Read the model definition and answer for the solid it produces. Units are mm, in the model's axes. A direction names the side the tool comes from. Round coordinates to 2 decimals unless told otherwise and drop trailing zeros. Write each loop counter-clockwise with the first axis right and the second up, starting at its lowest first coordinate (ties: lowest second). Pieces come first, ordered by that corner, then holes. Notation, with made-up numbers: (-5, 48.25) -> (7, 48.25) arc R9 cw to (7, 54.25) -> close; hole circle Ø6 at (37, 13.5). An arc over 180 degrees is marked (long way). Return JSON: item names as keys, results as strings. Group by question number.
(1) The mould has two halves that part along Z. Classify faces 1 (the flat face through (0, -152.4, 5)), 2 (the flat face through (-6.096, -75, -50)), 3 (the cylindrical face through (0.219, -129.486, -143.179)): released by +Z, released by -Z, zero draft, split by the parting line, or undercut.
(2) A cutting plane is placed at C-C on x = -21. Give the vertices of the cut face in (y, z).
(3) For faces 4 (the flat face through (0, -75, 0.191)), 5 (the flat face through (15.621, -58, -54)), 6 (the cylindrical face through (0.114, -131.979, -82.357)), 7 (the flat face through (0, 0, 5)), 8 (the flat face through (-15.621, -58, -52)), determine the directions among +Z, -Z, +X, -X, +Y, -Y from which every point of the face is accessible in a straight line to the end or side of a thin tool.
(4) A cutting plane is placed at D-D on y = -130. Give the vertices of the cut face in (x, z), then the cut area to 3 significant figures.
(5) Given pin 1 (1.5 mm diameter, centred on x = -10.5, y = -62.5, fed in from +Z); pin 2 (4 mm diameter, centred on x = 20, y = -24, fed in from +Z); pin 3 (8 mm diameter, centred on x = -19, z = -138.5, fed in from +Y); pin 4 (15 mm diameter, centred on x = 0, z = 38.29, fed in from -Y), each flat-ended and moving along its own axis, determine where each tip first touches the part or whether it passes through.
(6) Straight lines are drawn through the part: line 1 (Y direction, x = 7, z = 16.5); line 2 (X direction, y = -89, z = -46); line 3 (Z direction, x = 6, y = -76). For each, find the intervals that lie inside material, in ascending order.
(7) A cutting plane is placed at B-B on x = -10. State how many separate pieces and enclosed holes the cut face has, then the cut area to 3 significant figures.
(8) A cutting plane is placed at A-A on z = -41.5. Give the vertices of the cut face in (x, y).
```python
from build123d import *

# Parameters (mm, degrees)
F0_R          = 12.7
F1_DEPTH      = 152.4
F2_R          = 76.19999
F3_W          = 101.6
F3_H          = 56.6531687857
F4_DEPTH      = 41.022
F4_DEPTH_BACK = 25.4
F6_DEPTH      = 152.401
F3_H_2        = 18.0714114576
F7_DEPTH      = 41.022
F3_R          = 38.1
F8_DEPTH      = 41.022


# Not quite as in the source:
# - a fillet or chamfer is up to 0.001 mm smaller than in the source, because OpenCascade refuses the exact size
# - a feature names something its author has since deleted; it is built from what else it names


with BuildPart() as f1:
    # F0 (on Front) → F1 (new body)
    with BuildSketch(Plane.XZ):
        with BuildLine():
            ThreePointArc((15.621, 18.2628701244), (22.8246949596, 27.1472538948), (25.4, 38.2914586668))
            ThreePointArc((25.4, 38.2914586668), (-11.144204772, 61.1161536264), (-15.621, 18.2628701244))
            ThreePointArc((-15.621, 18.2628701244), (0, 12.8914586668), (15.621, 18.2628701244))
        make_face()
        with Locations((0, 38.2914586668)):
            Circle(F0_R, mode=Mode.SUBTRACT)
        with BuildLine():
            ThreePointArc((15.621, 18.2628701244), (0, 12.8914586668), (-15.621, 18.2628701244))
            Line((-15.621, 18.2628701244), (-15.621, -164.9085413332))
            Line((-15.621, -164.9085413332), (15.621, -164.9085413332))
            Line((15.621, -164.9085413332), (15.621, 18.2628701244))
        make_face()
    extrude(amount=F1_DEPTH)

    # F2 (radius 76.2 in the source; OpenCascade refuses exactly that, so slightly less here)
    f2_edges = [f1.edges().sort_by_distance(p)[0] for p in [
        (0, -152.4, -164.908541),
        (0, 0, -164.908541),
    ]]
    fillet(f2_edges, radius=F2_R)

    # F3 (on face) → F4 (cut, two sides)
    with BuildSketch(Plane(origin=(-15.621, 0, 0), x_dir=(0, -1, 0), z_dir=(-1, 0, 0))) as f4_sk:
        with Locations((76.2, 46.5894545172)):
            Rectangle(F3_W, F3_H)
    extrude(amount=-F4_DEPTH, mode=Mode.SUBTRACT)
    extrude(f4_sk.sketch, amount=F4_DEPTH_BACK, mode=Mode.SUBTRACT)

    # F5 (on Front) → F6 (cut, through all)
    with BuildSketch(Plane.XZ):
        with BuildLine():
            ThreePointArc((6.604, -25.2085413332), (0.254, -18.8585413332), (-6.096, -25.2085413332))
            Line((-6.096, -25.2085413332), (-6.096, -76.0085413332))
            ThreePointArc((-6.096, -76.0085413332), (0.254, -82.3585413332), (6.604, -76.0085413332))
            Line((6.604, -76.0085413332), (6.604, -25.2085413332))
        make_face()
    extrude(amount=F6_DEPTH, mode=Mode.SUBTRACT)

    # F3 (on face) → F7 (cut, through all)
    with BuildSketch(Plane(origin=(-15.621, 0, 0), x_dir=(0, -1, 0), z_dir=(-1, 0, 0))):
        with Locations((76.2, 9.2271643956)):
            Rectangle(F3_W, F3_H_2)
    extrude(amount=-F7_DEPTH, mode=Mode.SUBTRACT)

    # F3 (on face) → F8 (cut, through all)
    with BuildSketch(Plane(origin=(-15.621, 0, 0), x_dir=(0, -1, 0), z_dir=(-1, 0, 0))):
        with Locations((76.2, -88.7085413332)):
            Circle(F3_R)
    extrude(amount=-F8_DEPTH, mode=Mode.SUBTRACT)


solid = f1.part
```
Checks:
{
 "1": {"face 1": "zero draft", "face 2": "undercut", "face 3": "released by -Z"},
 "2": {"outline": "(-152.4, 24) -> (-127, 24) -> (-127, 52.58) -> (-152.4, 52.58) -> close; (-25.4, 24) -> (0, 24) -> (0, 52.58) -> (-25.4, 52.58) -> close"},
 "3": {"face 4": "+Z, +X, -X", "face 5": "-Z, +X, +Y, -Y", "face 6": "+Y, -Y", "face 7": "+Z, -Z, +X, -X, +Y", "face 8": "-Z, -X, +Y, -Y"},
 "4": {"outline": "(-15.62, -142.67) -> (15.62, -142.67) -> (15.62, 18.26) arc R25.4 ccw (long way) to (-15.62, 18.26) -> close; hole circle Ø25.4 at (0, 38.29); hole (-6.1, -76.01) arc R6.35 ccw to (6.6, -76.01) -> (6.6, -25.21) arc R6.35 ccw to (-6.1, -25.21) -> close", "area": "5,660 mm^2"},
 "5": {"pin 1": "stops at z = 0.19", "pin 2": "stops at z = 56.21", "pin 3": "stops at y = -16.74", "pin 4": "passes through"},
 "6": {"line 1": "y = -152.4 to -127, -25.4 to 0", "line 2": "x = -15.62 to -6.1, 6.6 to 15.62", "line 3": "z = -164.91 to -126.81, -22.51 to 0.19"},
 "7": {"separate pieces": "3", "enclosed holes": "1", "area": "20,400 mm^2"},
 "8": {"outline": "(-15.62, -152.4) -> (-6.1, -152.4) -> (-6.1, 0) -> (-15.62, 0) -> close; (6.6, -152.4) -> (15.62, -152.4) -> (15.62, 0) -> (6.6, 0) -> close"}
}
